Geometry check sheet. Reference: drawing and pictorial views, mm from the part's lowest x, y, z. Round coordinates to 2 decimals unless told otherwise and drop trailing zeros. Write each loop counter-clockwise with the first axis right and the second up, starting at its lowest first coordinate (ties: lowest second). Pieces come first, ordered by that corner, then holes. Notation, with made-up numbers: M 87,-14 L 91,-14 A23 cw 91,2 Z; hole C 7,64.5 d5. An arc over 180 degrees is marked long. Put each result on its own line as item: value. Start each with the question number.
(1) Material ranges on probe 1 along Y at (x, z) = (9, 4); probe 2 along X at (y, z) = (43, 4); probe 3 along Y at (x, z) = (5.5, 2.5), recorded low to high.
(2) Gauge pin test, flat ends, axial feed: pin 1 (1 mm diameter, centred on x = 25, z = 1.5, fed in from +Y); pin 2 (4 mm diameter, centred on x = 7.5, z = 1.5, fed in from -Y); pin 3 (3 mm diameter, centred on x = 7.5, y = 16.5, fed in from -Z). Record the tip position at first contact, or that the pin passes through.
(3) Section check C-C on x = 10.5. Record the cut outline in (y, z).
(4) Section check A-A on z = 3.5. Record the cut outline in (x, y) (3 decimals).
(5) Section check B-B on y = 48.5. Record the cut outline in (x, z), then the cut area to 3 significant figures.
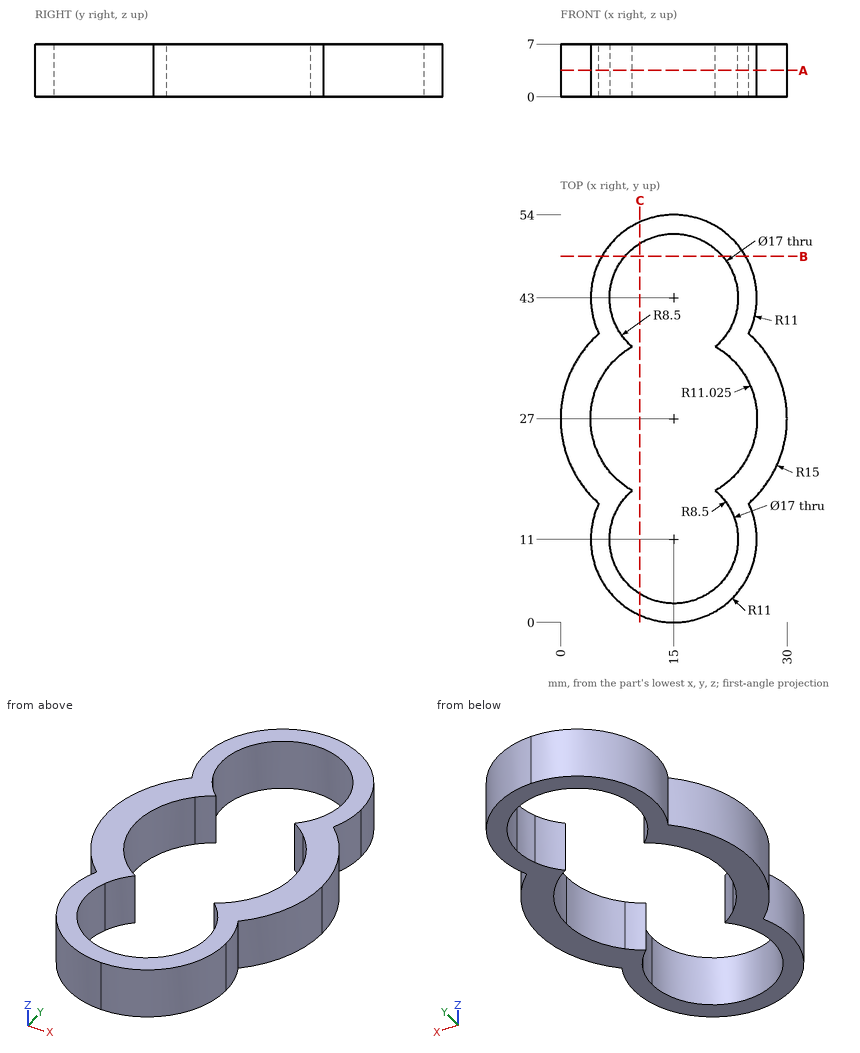
Answers follow:
1. probe 1: y = 1.78 to 4.98, 17.02 to 17.75, 36.25 to 36.98, 49.02 to 52.22
1. probe 2: x = 4 to 6.5, 23.5 to 26
1. probe 3: y = 5.45 to 21.41, 32.59 to 48.55
2. pin 1: stops at y = 48.55
2. pin 2: stops at y = 1.47
2. pin 3: stops at z = 0
3. outline: M 0.96,0 L 3.79,0 L 3.79,7 L 0.96,7 Z; M 50.21,0 L 53.04,0 L 53.04,7 L 50.21,7 Z
4. outline: M 5.078,15.75 A11 ccw long 24.922,15.75 A15 ccw 24.922,38.25 A11 ccw long 5.078,38.25 A15 ccw Z; hole M 9.475,17.459 A8.5 ccw long 20.525,17.459 A11.025 ccw 20.525,36.541 A8.5 ccw long 9.475,36.541 A11.025 ccw Z
5. outline: M 5.47,0 L 8.52,0 L 8.52,7 L 5.47,7 Z; M 21.48,0 L 24.53,0 L 24.53,7 L 21.48,7 Z
5. area: 42.6 mm^2
